```python
from build123d import *

# Parameters (mm, degrees)
F0_R             = 11
F1_DEPTH         = 3.5
F2_SIZE          = 1
F6_R             = 1
F7_DEPTH         = 7
F7_COPIES_COUNT  = 8
F9_R             = 1
F10_DEPTH        = 7
F10_COPIES_COUNT = 8


# Not quite as in the source:
# - a pattern or mirror of a feature is missing from the dataset's text; its kind, count and spacing are read off the source's solid


with BuildPart() as f1:
    # F0 (on Top) → F1 (new body, symmetric)
    with BuildSketch(Plane.XY):
        with BuildLine():
            ThreePointArc((12.0104759307, 4.9747832032), (12.750219353, 2.5361203541), (13, 0))
            ThreePointArc((13, 0), (12.750219353, -2.5361203541), (12.0104759307, -4.9747832032))
            ThreePointArc((12.0104759307, -4.9747832032), (12.0107097924, -4.9749394725), (12.0109436454, -4.9750957548))
            ThreePointArc((12.0109436454, -4.9750957548), (18.0724560365, 0), (12.0109436454, 4.9750957548))
            ThreePointArc((12.0109436454, 4.9750957548), (12.0107097924, 4.9749394725), (12.0104759307, 4.9747832032))
        make_face()
        with BuildLine():
            ThreePointArc((12.0103919138, 4.974986038), (12.0104339226, 4.9748846207), (12.0104759307, 4.9747832032))
            ThreePointArc((12.0104759307, 4.9747832032), (12.0107097924, 4.9749394725), (12.0109436454, 4.9750957548))
            ThreePointArc((12.0109436454, 4.9750957548), (12.0106677781, 4.975040904), (12.0103919138, 4.974986038))
        make_face()
        with BuildLine():
            ThreePointArc((12.0109436454, -4.9750957548), (12.0107097924, -4.9749394725), (12.0104759307, -4.9747832032))
            ThreePointArc((12.0104759307, -4.9747832032), (12.0104339226, -4.9748846207), (12.0103919138, -4.974986038))
            ThreePointArc((12.0103919138, -4.974986038), (12.0106677781, -4.975040904), (12.0109436454, -4.9750957548))
        make_face()
        with BuildLine():
            ThreePointArc((4.974986038, 12.0103919138), (9.1923881554, 9.1923881554), (12.0103919138, 4.974986038))
            ThreePointArc((12.0103919138, 4.974986038), (12.0106677781, 4.975040904), (12.0109436454, 4.9750957548))
            ThreePointArc((12.0109436454, 4.9750957548), (12.7791562161, 12.7791562161), (4.9750957548, 12.0109436454))
            ThreePointArc((4.9750957548, 12.0109436454), (4.975040904, 12.0106677781), (4.974986038, 12.0103919138))
        make_face()
        with BuildLine():
            ThreePointArc((12.0109436454, -4.9750957548), (12.0106677781, -4.975040904), (12.0103919138, -4.974986038))
            ThreePointArc((12.0103919138, -4.974986038), (9.1923881554, -9.1923881554), (4.974986038, -12.0103919138))
            ThreePointArc((4.974986038, -12.0103919138), (4.975040904, -12.0106677781), (4.9750957548, -12.0109436454))
            ThreePointArc((4.9750957548, -12.0109436454), (12.7791562161, -12.7791562161), (12.0109436454, -4.9750957548))
        make_face()
        with BuildLine():
            ThreePointArc((4.9747832032, 12.0104759307), (4.9748846207, 12.0104339226), (4.974986038, 12.0103919138))
            ThreePointArc((4.974986038, 12.0103919138), (4.975040904, 12.0106677781), (4.9750957548, 12.0109436454))
            ThreePointArc((4.9750957548, 12.0109436454), (4.9749394725, 12.0107097924), (4.9747832032, 12.0104759307))
        make_face()
        with BuildLine():
            ThreePointArc((4.9747832032, 12.0104759307), (4.9749394725, 12.0107097924), (4.9750957548, 12.0109436454))
            ThreePointArc((4.9750957548, 12.0109436454), (0, 18.0724560365), (-4.9750957548, 12.0109436454))
            ThreePointArc((-4.9750957548, 12.0109436454), (-4.9749394725, 12.0107097924), (-4.9747832032, 12.0104759307))
            ThreePointArc((-4.9747832032, 12.0104759307), (0, 13), (4.9747832032, 12.0104759307))
        make_face()
        with BuildLine():
            ThreePointArc((4.9750957548, -12.0109436454), (4.975040904, -12.0106677781), (4.974986038, -12.0103919138))
            ThreePointArc((4.974986038, -12.0103919138), (4.9748846207, -12.0104339226), (4.9747832032, -12.0104759307))
            ThreePointArc((4.9747832032, -12.0104759307), (4.9749394725, -12.0107097924), (4.9750957548, -12.0109436454))
        make_face()
        with BuildLine():
            ThreePointArc((-4.9750957548, -12.0109436454), (0, -18.0724560365), (4.9750957548, -12.0109436454))
            ThreePointArc((4.9750957548, -12.0109436454), (4.9749394725, -12.0107097924), (4.9747832032, -12.0104759307))
            ThreePointArc((4.9747832032, -12.0104759307), (0, -13), (-4.9747832032, -12.0104759307))
            ThreePointArc((-4.9747832032, -12.0104759307), (-4.9749394725, -12.0107097924), (-4.9750957548, -12.0109436454))
        make_face()
        with BuildLine():
            ThreePointArc((-4.9747832032, 12.0104759307), (-4.9749394725, 12.0107097924), (-4.9750957548, 12.0109436454))
            ThreePointArc((-4.9750957548, 12.0109436454), (-4.975040904, 12.0106677781), (-4.974986038, 12.0103919138))
            ThreePointArc((-4.974986038, 12.0103919138), (-4.9748846207, 12.0104339226), (-4.9747832032, 12.0104759307))
        make_face()
        with BuildLine():
            ThreePointArc((-4.974986038, 12.0103919138), (-4.975040904, 12.0106677781), (-4.9750957548, 12.0109436454))
            ThreePointArc((-4.9750957548, 12.0109436454), (-12.7791562161, 12.7791562161), (-12.0109436454, 4.9750957548))
            ThreePointArc((-12.0109436454, 4.9750957548), (-12.0106677781, 4.975040904), (-12.0103919138, 4.974986038))
            ThreePointArc((-12.0103919138, 4.974986038), (-9.1923881554, 9.1923881554), (-4.974986038, 12.0103919138))
        make_face()
        with BuildLine():
            ThreePointArc((-4.974986038, -12.0103919138), (-4.975040904, -12.0106677781), (-4.9750957548, -12.0109436454))
            ThreePointArc((-4.9750957548, -12.0109436454), (-4.9749394725, -12.0107097924), (-4.9747832032, -12.0104759307))
            ThreePointArc((-4.9747832032, -12.0104759307), (-4.9748846207, -12.0104339226), (-4.974986038, -12.0103919138))
        make_face()
        with BuildLine():
            ThreePointArc((-12.0109436454, -4.9750957548), (-12.7791562161, -12.7791562161), (-4.9750957548, -12.0109436454))
            ThreePointArc((-4.9750957548, -12.0109436454), (-4.975040904, -12.0106677781), (-4.974986038, -12.0103919138))
            ThreePointArc((-4.974986038, -12.0103919138), (-9.1923881554, -9.1923881554), (-12.0103919138, -4.974986038))
            ThreePointArc((-12.0103919138, -4.974986038), (-12.0106677781, -4.975040904), (-12.0109436454, -4.9750957548))
        make_face()
        with BuildLine():
            ThreePointArc((-12.0103919138, 4.974986038), (-12.0106677781, 4.975040904), (-12.0109436454, 4.9750957548))
            ThreePointArc((-12.0109436454, 4.9750957548), (-12.0107097924, 4.9749394725), (-12.0104759307, 4.9747832032))
            ThreePointArc((-12.0104759307, 4.9747832032), (-12.0104339226, 4.9748846207), (-12.0103919138, 4.974986038))
        make_face()
        with BuildLine():
            ThreePointArc((-12.0104759307, 4.9747832032), (-12.0107097924, 4.9749394725), (-12.0109436454, 4.9750957548))
            ThreePointArc((-12.0109436454, 4.9750957548), (-18.0724560365, 0), (-12.0109436454, -4.9750957548))
            ThreePointArc((-12.0109436454, -4.9750957548), (-12.0107097924, -4.9749394725), (-12.0104759307, -4.9747832032))
            ThreePointArc((-12.0104759307, -4.9747832032), (-13, 0), (-12.0104759307, 4.9747832032))
        make_face()
        with BuildLine():
            ThreePointArc((-12.0104759307, -4.9747832032), (-12.0107097924, -4.9749394725), (-12.0109436454, -4.9750957548))
            ThreePointArc((-12.0109436454, -4.9750957548), (-12.0106677781, -4.975040904), (-12.0103919138, -4.974986038))
            ThreePointArc((-12.0103919138, -4.974986038), (-12.0104339226, -4.9748846207), (-12.0104759307, -4.9747832032))
        make_face()
        with BuildLine():
            ThreePointArc((12.0104759307, -4.9747832032), (12.750219353, -2.5361203541), (13, 0))
            ThreePointArc((13, 0), (12.750219353, 2.5361203541), (12.0104759307, 4.9747832032))
            ThreePointArc((12.0104759307, 4.9747832032), (12.0104339226, 4.9748846207), (12.0103919138, 4.974986038))
            ThreePointArc((12.0103919138, 4.974986038), (9.1923881554, 9.1923881554), (4.974986038, 12.0103919138))
            ThreePointArc((4.974986038, 12.0103919138), (4.9748846207, 12.0104339226), (4.9747832032, 12.0104759307))
            ThreePointArc((4.9747832032, 12.0104759307), (0, 13), (-4.9747832032, 12.0104759307))
            ThreePointArc((-4.9747832032, 12.0104759307), (-4.9748846207, 12.0104339226), (-4.974986038, 12.0103919138))
            ThreePointArc((-4.974986038, 12.0103919138), (-9.1923881554, 9.1923881554), (-12.0103919138, 4.974986038))
            ThreePointArc((-12.0103919138, 4.974986038), (-12.0104339226, 4.9748846207), (-12.0104759307, 4.9747832032))
            ThreePointArc((-12.0104759307, 4.9747832032), (-13, 0), (-12.0104759307, -4.9747832032))
            ThreePointArc((-12.0104759307, -4.9747832032), (-12.0104339226, -4.9748846207), (-12.0103919138, -4.974986038))
            ThreePointArc((-12.0103919138, -4.974986038), (-9.1923881554, -9.1923881554), (-4.974986038, -12.0103919138))
            ThreePointArc((-4.974986038, -12.0103919138), (-4.9748846207, -12.0104339226), (-4.9747832032, -12.0104759307))
            ThreePointArc((-4.9747832032, -12.0104759307), (0, -13), (4.9747832032, -12.0104759307))
            ThreePointArc((4.9747832032, -12.0104759307), (4.9748846207, -12.0104339226), (4.974986038, -12.0103919138))
            ThreePointArc((4.974986038, -12.0103919138), (9.1923881554, -9.1923881554), (12.0103919138, -4.974986038))
            ThreePointArc((12.0103919138, -4.974986038), (12.0104339226, -4.9748846207), (12.0104759307, -4.9747832032))
        make_face()
        Circle(F0_R, mode=Mode.SUBTRACT)
    extrude(amount=F1_DEPTH, both=True)

    # F2
    f2_edges = [f1.edges().sort_by_distance(p)[0] for p in [
        (-11, 0, 3.5),
        (-11, 0, -3.5),
    ]]
    chamfer(f2_edges, length=F2_SIZE)

    # F6 (on line) → F7 (cut)
    with BuildSketch(Plane(origin=(-5.2779168675, 19.6974539077, 0), x_dir=(-0.9659258263, -0.2588190451, 0), z_dir=(-0.2588190451, 0.9659258263, 0))):
        with Locations((6, 0)):
            Circle(F6_R)
    f7 = extrude(amount=-F7_DEPTH, mode=Mode.SUBTRACT)

    # F7_copies: F7 ×8 about axis
    f7_copies_axis = Axis((0, 0, 0), (0, 0, 1))
    for i in range(1, F7_COPIES_COUNT):
        add(f7.rotate(f7_copies_axis, i * 360 / F7_COPIES_COUNT), mode=Mode.SUBTRACT)

    # F9 (on line) → F10 (cut)
    with BuildSketch(Plane(origin=(-19.6974539077, 5.2779168675, 0), x_dir=(-0.2588190451, -0.9659258263, 0), z_dir=(-0.9659258263, 0.2588190451, 0))):
        with Locations((-6, 0)):
            Circle(F9_R)
    f10 = extrude(amount=-F10_DEPTH, mode=Mode.SUBTRACT)

    # F10_copies: F10 ×8 about axis
    f10_copies_axis = Axis((0, 0, 0), (0, 0, 1))
    for i in range(1, F10_COPIES_COUNT):
        add(f10.rotate(f10_copies_axis, i * 360 / F10_COPIES_COUNT), mode=Mode.SUBTRACT)


solid = f1.part
```
Verification items for the finished model (mm, model axes). Round coordinates to 2 decimals unless told otherwise and drop trailing zeros. Order: outer loops, then holes, each group sorted by start corner. A loop starts at its lowest first (then second) coordinate and runs counter-clockwise, first axis right, second up. Notation, with made-up numbers: (78, 84) - (120, 84) arc R12 cw to (120, 99) - close; hole circle Ø7 at (-10, 35). An arc over 180 degrees is marked (long way). Use CSV: the item, a comma, the result in double quotes. Start each with the question number.
1) Section check C-C, the plane y = -13. State how many separate pieces and enclosed holes the cut face has, plus the area to 3 significant figures.
2) Go/stop test with flat-tipped pins: P1, Ø2, axis at x = -3, z = -1, coming from the -Y side; P2, Ø3, axis at y = 12, z = 2.5, coming from the +X side; P3, Ø1.5, axis at y = -3, z = 2, coming from the +X side. Record where each tip stops, or that it passes through.
3) Section check A-A, the plane x = 0. Record the cut outline in (y, z), plus the area to 3 significant figures.
4) Section check D-D, the plane z = 3. Record the cut outline in (x, y).
5) Thickness scan on L1, parallel to Y at x = -12.5, z = 0.25; L2, parallel to Y at x = 2, z = -2; L3, parallel to Y at x = -13, z = 3.25. Record the ranges inside material, lowest first.
6) Section check B-B, the plane z = -2. Record the cut outline in (x, y).
Answers:
1,separate pieces,"3"
1,enclosed holes,"2"
1,area,"158 mm²"
2,P1,"stops at y = -17.66"
2,P2,"stops at x = 14.09"
2,P3,"stops at x = 17.55"
3,outline,"(-18.07, -3.5) - (-12, -3.5) - (-11, -2.5) - (-11, 2.5) - (-12, 3.5) - (-18.07, 3.5) - close; (11, -2.5) - (12, -3.5) - (18.07, -3.5) - (18.07, 3.5) - (12, 3.5) - (11, 2.5) - close"
3,area,"97.0 mm²"
4,outline,"(-12.01, -4.98) arc R5.07 ccw (long way) to (-4.98, -12.01) arc R5.07 ccw (long way) to (4.98, -12.01) arc R5.07 ccw (long way) to (12.01, -4.98) arc R5.07 ccw (long way) to (12.01, 4.98) arc R5.07 ccw (long way) to (4.98, 12.01) arc R5.07 ccw (long way) to (-4.98, 12.01) arc R5.07 ccw (long way) to (-12.01, 4.98) arc R5.07 ccw (long way) to start; hole circle Ø23 at (0, 0)"
5,L1,"y = -13.04 to -10.56, -8.56 to -5.35, -5.05 to 5.05, 5.35 to 8.56, 10.56 to 13.04"
5,L2,"y = -17.66 to -10.82, 10.82 to 17.66"
5,L3,"y = -12.54 to -5.84, -5.07 to 5.07, 5.84 to 12.54"
6,outline,"(-12.01, -4.98) arc R5.07 ccw (long way) to (-4.98, -12.01) arc R5.07 ccw (long way) to (4.98, -12.01) arc R5.07 ccw (long way) to (12.01, -4.98) arc R5.07 ccw (long way) to (12.01, 4.98) arc R5.07 ccw (long way) to (4.98, 12.01) arc R5.07 ccw (long way) to (-4.98, 12.01) arc R5.07 ccw (long way) to (-12.01, 4.98) arc R5.07 ccw (long way) to start; hole circle Ø22 at (0, 0)"
